from build123d import *

# Parameters (mm, degrees)
SKETCH_1_W               = 98
SKETCH_1_H               = 119
SKETCH_1_R               = 1.9
EXTRUDE_1_DEPTH          = 4
SKETCH_2_W               = 74
SKETCH_2_H               = 119
SKETCH_2_W_2             = 68
SKETCH_2_H_2             = 113
EXTRUDE_1_2_DEPTH        = 20
FILLET_1_R               = 5
CHAMFER_1_SIZE           = 2
CUT_EXTRUDE_1_DEPTH      = 80.631965943
CUT_EXTRUDE_1_DEPTH_BACK = 80.631965943
SKETCH_3_R               = 6.5
FILLET_2_R               = 5


with BuildPart() as part:
    # Эскиз1 → Extrude 1 (new body)
    with BuildSketch(Plane(origin=(0, 0, 0), x_dir=(1, 0, 0), z_dir=(0, 1, 0))):
        Rectangle(SKETCH_1_W, SKETCH_1_H)
        with Locations(Location((-45, 45, 0), (0, 0, 270))):
            Circle(SKETCH_1_R, mode=Mode.SUBTRACT)
        with Locations(Location((45, 45, 0), (0, 0, 90))):
            Circle(SKETCH_1_R, mode=Mode.SUBTRACT)
        with Locations(Location((45, -45, 0), (0, 0, 270))):
            Circle(SKETCH_1_R, mode=Mode.SUBTRACT)
        with Locations(Location((-45, -45, 0), (0, 0, 90))):
            Circle(SKETCH_1_R, mode=Mode.SUBTRACT)
    extrude(amount=EXTRUDE_1_DEPTH)

    # Эскиз2 → Extrude 1 2 (add)
    with BuildSketch(Plane(origin=(0, 4, 0), x_dir=(1, 0, 0), z_dir=(0, 1, 0))):
        Rectangle(SKETCH_2_W, SKETCH_2_H)
        Rectangle(SKETCH_2_W_2, SKETCH_2_H_2, mode=Mode.SUBTRACT)
    extrude(amount=EXTRUDE_1_2_DEPTH)

    # Скругление1
    fillet_1_edges = [part.edges().sort_by_distance(p)[0] for p in [
        (37, 4, 0),
        (-37, 4, 0),
    ]]
    fillet(fillet_1_edges, radius=FILLET_1_R)

    # Фаска1
    chamfer_1_edges = [part.edges().sort_by_distance(p)[0] for p in [
        (-49, 0, 0),
        (49, 0, 0),
    ]]
    chamfer(chamfer_1_edges, length=CHAMFER_1_SIZE)

    # Эскиз3 → Вырез-Вытянуть1 (cut, two sides: drawn at the far end of the back side and taken through both)
    with BuildSketch(Plane(origin=(0, 4, 0), x_dir=(1, 0, 0), z_dir=(0, 1, 0)).offset(-CUT_EXTRUDE_1_DEPTH_BACK)):
        with Locations((44, 59.5)):
            Circle(SKETCH_3_R)
        with Locations((-44, 59.5)):
            Circle(SKETCH_3_R)
        with Locations((44, -59.5)):
            Circle(SKETCH_3_R)
        with Locations((-44, -59.5)):
            Circle(SKETCH_3_R)
    extrude(amount=CUT_EXTRUDE_1_DEPTH + CUT_EXTRUDE_1_DEPTH_BACK, mode=Mode.SUBTRACT)

    # Скругление2
    fillet_2_edges = [part.edges().sort_by_distance(p)[0] for p in [
        (-49, 3, 55.346688069),
        (49, 3, 55.346688069),
        (-49, 3, -55.346688069),
        (49, 3, -55.346688069),
    ]]
    fillet(fillet_2_edges, radius=FILLET_2_R)


solid = part.part
The listing builds one solid part. Answer for the finished solid, in the listing's coordinates (mm). A direction names the side the tool comes from. Coordinates: 2 decimals unless noted, no trailing zeros. Write each loop counter-clockwise with the first axis right and the second up, starting at its lowest first coordinate (ties: lowest second). Pieces come first, ordered by that corner, then holes. Notation, with made-up numbers: M -26,15 L -8,15 A29 ccw -8,54 Z; hole C -22,37 d5. An arc over 180 degrees is marked long. Put each result on its own line as item: value. Start each with the question number.
1. A cutting plane is placed at B-B on x = -24.5. Write down the section's boundary in (y, z), then the cut area to 3 significant figures.
2. Flat-ended cylindrical pins translate along their axes: P1, Ø3.5, axis at x = 46, z = -3.5, coming from the +Y side; P2, Ø4, axis at x = -1, z = -24.5, coming from the -Y side; P3, Ø6, axis at y = 13, z = 36, coming from the +X side; P4, Ø4.5, axis at y = 19, z = -22, coming from the -X side. Find the tip coordinate at first contact, or state that the pin passes through.
3. A cutting plane is placed at A-A on z = 45. Write down the section's boundary in (x, y), then the cut area to 3 significant figures.
4. A cutting plane is placed at D-D on z = 21.5. Write down the section's boundary in (x, y), then the cut area to 3 significant figures.
5. Which of the six approach directions +Z, -Z, +X, -X, +Y, -Y give full straight-line access (tool end or side, diameter ignored) to faces 4 (the flat face through (0, 14, -56.5)), 5 (the flat face through (37, 16, 1)), 6 (the flat face through (-37, 16, 1)), 7 (the cylindrical face through (-38.72, 2.6, -55.71))?
6. Consider line 1 (X direction, y = 2.8, z = 45); line 2 (Z direction, x = -10, y = 15.75); line 3 (X direction, y = 16.25, z = -16). Determine where each line is inside the solid, lowest interval first. Write a range as from..to.
7. For a pull along Z with two mould halves and no side action, classify faces 1 (the flat face through (-34, 14, 1)), 2 (the cylindrical face through (-47, 2, 52)), 3 (the flat face through (-36, 24, 0)) as pulls with the +Z half, pulls with the -Z half, needs draft (parallel to the pull), parting line crosses it, or undercut.
8. A cutting plane is placed at C-C on y = 10.25. Write down the section's boundary in (x, z).
Resolved:
1. outline: M 0,-59.5 L 24,-59.5 L 24,-56.5 L 4,-56.5 L 4,56.5 L 24,56.5 L 24,59.5 L 0,59.5 Z
1. area: 596 mm2
2. P1: stops at y = 4
2. P2: stops at y = 0
2. P3: stops at x = 37
2. P4: stops at x = -37
3. outline: M -49,2 L -47,0 L -46.9,0 L -46.9,4 L -49,4 Z; M -43.1,0 L 43.1,0 L 43.1,4 L 42,4 A5 cw 37,9 L 37,24 L 34,24 L 34,4 L -34,4 L -34,24 L -37,24 L -37,9 A5 cw -42,4 L -43.1,4 Z; M 46.9,0 L 47,0 L 49,2 L 49,4 L 46.9,4 Z
3. area: 488 mm2
4. outline: M -49,2 L -47,0 L 47,0 L 49,2 L 49,4 L 42,4 A5 cw 37,9 L 37,24 L 34,24 L 34,4 L -34,4 L -34,24 L -37,24 L -37,9 A5 cw -42,4 L -49,4 Z
4. area: 519 mm2
5. face 4: +Y
5. face 5: +Z, -Z, +X, +Y
5. face 6: +Z, -Z, -X, +Y
5. face 7: -Z, -X, +Y, -Y
6. line 1: x = -49..-46.9, -43.1..43.1, 46.9..49
6. line 2: z = -59.5..-56.5, 56.5..59.5
6. line 3: x = -37..-34, 34..37
7. face 1: undercut
7. face 2: pulls with the +Z half
7. face 3: needs draft
8. outline: M -37,-59.5 L 37,-59.5 L 37,59.5 L -37,59.5 Z; hole M -34,-56.5 L 34,-56.5 L 34,56.5 L -34,56.5 Z
